Autodesk Inventor part; units mm, degrees
ref_plane "YZ Plane" through (0, 0, 0) normal (1, 0, 0) x (0, 1, 0)
ref_plane "XZ Plane" through (0, 0, 0) normal (0, 1, 0) x (-1, 0, 0)
ref_plane "XY Plane" through (0, 0, 0) normal (0, 0, 1) x (1, 0, 0)
sketch "Sketch1" plane through (0, 0, 0) normal (0, 0, 1) x (1, 0, 0)
  line L0 (0, 7) -> (0, -7)
  line L1 (-7, 0) -> (7, 0)
  line L2 (5, -5) -> (-5, -5)
  line L3 (-5, -5) -> (-5, 5)
  line L4 (-5, 5) -> (5, 5)
  line L5 (5, 5) -> (5, -5)
  line L6 (5, -5) -> (-5, 5) construction
  line L7 (-5, -5) -> (5, 5) construction
  point P0 (0, 0)
  dimension "d0" = 10
  dimension "d1" = 10
extrude "Extrusion1" add sketch "Sketch1" along normal blind 25.4
chamfer "Chamfer1" distance 9.5 angle 45 1 edges at (0, 5, 25.4)
properties part number "ADAFRUIT 1512 LOCK SOLENOID PLUNGER"
Could you check a few things on this model? Use its own coordinates, in mm. Coordinates: 2 decimals unless noted, no trailing zeros. Loops run counter-clockwise (first coordinate to the right, second up) from the corner with the lowest first, then second, coordinate; pieces in that order, holes last.
1. I need wall thicknesses on L1, parallel to Y at x = -1.5, z = 16; L2, parallel to Z at x = -3.75, y = 3.25; L3, parallel to Y at x = -3, z = 22.25. Which ranges of each line are inside material? Lowest first, please.
2. Imagine slicing it at C-C (y = -0.75). Please give me the cut outline in (x, z).
3. Imagine slicing it at B-B (y = 4.25). Please give me the cut outline in (x, z), and give its area (4 significant figures).
4. Imagine slicing it at A-A (x = 2). Please give me the cut outline in (y, z), and give its area (3 significant figures).
5. For P1, Ø1.5, axis at x = 2, y = -3, coming from the +Z side; P2, Ø4, axis at x = 2.5, y = -1, coming from the +Z side; P3, Ø3, axis at x = 3, z = 17.5, coming from the +Y side, each with a flat end and sliding along its axis, tell me the tip position at first contact or that it passes through.
Computed values:
1. L1: y = -5 to 4.9
1. L2: z = 0 to 17.65
1. L3: y = -5 to -1.35
2. outline: (-5, 0) - (5, 0) - (5, 21.65) - (-5, 21.65) - close
3. outline: (-5, 0) - (5, 0) - (5, 16.65) - (-5, 16.65) - close
3. area: 166.5 mm2
4. outline: (-5, 0) - (5, 0) - (5, 15.9) - (-4.5, 25.4) - (-5, 25.4) - close
4. area: 209 mm2
5. P1: stops at z = 24.65
5. P2: stops at z = 23.9
5. P3: stops at y = 4.9
